Source: CAD feature listing. Evaluate the final solid. Frame: model axes, mm. Give positions to 0.01 mm unless a question says otherwise; leave off trailing zeros. Order: outer loops, then holes, each group sorted by start corner. A loop starts at its lowest first (then second) coordinate and runs counter-clockwise, first axis right, second up.
1) Section C-C, the plane y = 29. Return loops of the section in (x, z), plus the area to 3 significant figures.
2) First-contact query: P1, Ø1.5, axis at x = 3, y = 29, coming from the +Z side; P2, Ø10, axis at x = 14.5, y = -3, coming from the -Z side. Flat tips, straight axial feed; report the tip coordinate or a pass-through.
3) Material intervals for line 1 (X direction, y = -25, z = -0.9); line 2 (Y direction, x = -14, z = -1.4); line 3 (Y direction, x = -8, z = -0.15), sorted ascending.
4) Section A-A, the plane y = -13. Return loops of the section in (x, z).
5) Section D-D, the plane x = 16. Return loops of the section in (y, z), plus the area to 3 significant figures.
6) Section B-B, the plane x = 3. Return loops of the section in (y, z).
```python
from build123d import *

# Parameters (mm, degrees)
SKETCH_W     = 50
SKETCH_H     = 74
SKETCH_W_2   = 40
SKETCH_H_2   = 55
PAD_DEPTH    = 2
SKETCH001_W  = 25
SKETCH001_H  = 6
POCKET_DEPTH = 1.4
FILLET003_R  = 1
FILLET004_R  = 2
FILLET006_R  = 0.5


with BuildPart() as part:
    # Sketch → Pad (new body)
    with BuildSketch(Plane.XY):
        with Locations((0, 2.5)):
            Rectangle(SKETCH_W, SKETCH_H)
        Rectangle(SKETCH_W_2, SKETCH_H_2, mode=Mode.SUBTRACT)
    extrude(amount=-PAD_DEPTH)

    # Sketch001 → Pocket (cut)
    with BuildSketch(Plane.XY):
        with Locations((0, 30.5)):
            Rectangle(SKETCH001_W, SKETCH001_H)
    extrude(amount=-POCKET_DEPTH, mode=Mode.SUBTRACT)

    # Fillet003
    fillet003_edges = [part.edges().sort_by_distance(p)[0] for p in [
        (0, 33.5, -1.4),
    ]]
    fillet(fillet003_edges, radius=FILLET003_R)

    # Fillet004
    fillet004_edges = [part.edges().sort_by_distance(p)[0] for p in [
        (-25, -34.5, -1),
        (25, -34.5, -1),
        (-25, 39.5, -1),
        (25, 39.5, -1),
    ]]
    fillet(fillet004_edges, radius=FILLET004_R)

    # Fillet006
    fillet006_edges = [part.edges().sort_by_distance(p)[0] for p in [
        (-12.5, 30, -1.4),
        (-12.5, 33.207107, -1.107107),
        (-12.5, 33.5, -0.2),
    ]]
    fillet(fillet006_edges, radius=FILLET006_R)


solid = part.part
```
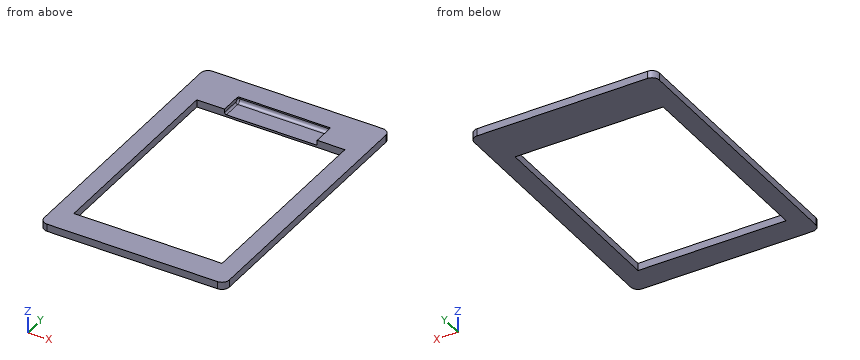
From the geometry:
1. outline: (-25, -2) - (25, -2) - (25, 0) - (12.5, 0) - (12.5, -1.4) - (-12, -1.4) arc R0.5 cw to (-12.5, -0.9) - (-12.5, 0) - (-25, 0) - close
1. area: 65.1 mm2
2. P1: stops at z = -1.4
2. P2: passes through
3. line 1: x = -25 to -20, 20 to 25
3. line 2: y = -34.5 to -27.5, 27.5 to 39.5
3. line 3: y = -34.5 to -27.5, 33.5 to 39.5
4. outline: (-25, -2) - (-20, -2) - (-20, 0) - (-25, 0) - close; (20, -2) - (25, -2) - (25, 0) - (20, 0) - close
5. outline: (-34.5, -2) - (-27.5, -2) - (-27.5, 0) - (-34.5, 0) - close; (27.5, -2) - (39.5, -2) - (39.5, 0) - (27.5, 0) - close
5. area: 38.0 mm2
6. outline: (-34.5, -2) - (-27.5, -2) - (-27.5, 0) - (-34.5, 0) - close; (27.5, -2) - (39.5, -2) - (39.5, 0) - (33.5, 0) - (33.5, -0.4) arc R1 cw to (32.5, -1.4) - (27.5, -1.4) - close
